Could you check a few things on this model? Use its own coordinates, in mm. A direction names the side the tool comes from. Coordinates: 2 decimals unless noted, no trailing zeros. Order: outer loops, then holes, each group sorted by start corner. A loop starts at its lowest first (then second) coordinate and runs counter-clockwise, first axis right, second up. Notation, with made-up numbers: (37, 35) -> (73, 35) arc R18 cw to (73, 56) -> close; hole circle Ø6 at (1, -24). An arc over 180 degrees is marked (long way). Put each result on its own line as item: value. Start each with the question number.
Q1. For faces 5 (the face through (41, 4, -52.5)), 6 (the face through (35, 60.5, -59)), which set-ups out of +Z, -Z, +X, -X, +Y, -Y let a thin tool reach every point of the face, with its end or its side?
Q2. We'd pull the mould along X, two halves only. Please class faces 1 (the face through (2, 4, -59)), 2 (the face through (33.226, 35.923, -53.514)), 3 (the face through (2.5, 5.8, -54)), 4 (the face through (1, -12, -62.5)): +X half, -X half, draft (parallel to the pull), parting line (faces both ways), or undercut.
Q3. If we section it at D-D (z = -58.75): Please give me the cut outline in (x, y).
Q4. Will these pins go through, and if not, where does the flat tip stop? pin 1 (1 mm diameter, centred on x = 28.5, y = 47.5, fed in from -Z); pin 2 (1.6 mm diameter, centred on x = 35, z = -54, fed in from -Y); pin 3 (0.6 mm diameter, centred on y = 2.5, z = -54, fed in from -X); pin 4 (3.5 mm diameter, centred on x = 35, y = 35, fed in from +Z).
Q5. Please list where these lines run through material, in increasing order: line 1 along Y through (x, z) = (47, -59.5); line 2 along X through (y, z) = (46, -57.5); line 3 along Z through (x, y) = (12, -24.5).
from build123d import *

# Parameters (mm, degrees)
SKETCH1_W             = 70
SKETCH1_H             = 115
BOSS_EXTRUDE1_DEPTH   = 10
CUT_EXTRUDE1_DEPTH    = 8
CHAMFER1_SIZE         = 4
SKETCH2_R             = 2
SKETCH2_W             = 10
SKETCH2_H             = 25
CUT_EXTRUDE2_DEPTH    = 8
BODY_MOVE_COPY1_ANGLE = 90


with BuildPart() as part:
    # Sketch1 → Boss-Extrude1 (new body)
    with BuildSketch(Plane(origin=(0, 0, 0), x_dir=(1, 0, 0), z_dir=(0, 1, 0))):
        with Locations((35, 57.5)):
            Rectangle(SKETCH1_W, SKETCH1_H)
    extrude(amount=BOSS_EXTRUDE1_DEPTH)

    # 3DSketch1 → Cut-Extrude1 (cut)
    with BuildSketch(Plane(origin=(2, 10, -2), x_dir=(0.51107539287715, 0, -0.8595358880206614), z_dir=(0, -1, 0))):
        Polygon((0, 0), (33.73097593, 56.729368609), (129.1394595, 0), (95.40848357, -56.729368609), align=None)
    extrude(amount=CUT_EXTRUDE1_DEPTH, mode=Mode.SUBTRACT)

    # Chamfer1
    chamfer1_edges = [part.edges().sort_by_distance(p)[0] for p in [
        (35, 0, -115),
        (70, 0, -57.5),
        (35, 0, 0),
        (0, 0, -57.5),
    ]]
    chamfer(chamfer1_edges, length=CHAMFER1_SIZE)

    # Sketch2 → Cut-Extrude2 (cut)
    with BuildSketch(Plane(origin=(0, 2, 0), x_dir=(1, 0, 0), z_dir=(0, 1, 0))):
        with Locations(Location((35, 87.5, 0), (0, 0, 270))):
            Circle(SKETCH2_R)
        with Locations(Location((35, 27.5, 0), (0, 0, 270))):
            Circle(SKETCH2_R)
        with Locations((35, 57.5)):
            Rectangle(SKETCH2_W, SKETCH2_H)
    extrude(amount=-CUT_EXTRUDE2_DEPTH, mode=Mode.SUBTRACT)


with BuildPart() as part_1:
    # Body-Move/Copy1: moved
    add(part.part.rotate(Axis((0, 5.000051539, -57.5), (-1, 0, 0)), BODY_MOVE_COPY1_ANGLE))


solid = part_1.part
The answers:
1. face 5: +Z, +X, -X, +Y, -Y
1. face 6: -Z
2. face 1: undercut
2. face 2: undercut
2. face 3: -X half
2. face 4: draft
3. outline: (0, -52.5) -> (70, -52.5) -> (70, 62.5) -> (0, 62.5) -> close; hole (2, -50.5) -> (68, -50.5) -> (68, 60.5) -> (2, 60.5) -> close
4. pin 1: z = -54.5
4. pin 2: y = -50.8
4. pin 3: x = 2.2
4. pin 4: through
5. line 1: -52.5 to -50.5, 60.5 to 62.5
5. line 2: 0 to 2, 68 to 70
5. line 3: -54.5 to -52.5
